Autodesk Inventor part; units mm, degrees
sketch "Skizze1" plane through (0, 0, 0) normal (0, 1, 0) x (-1, 0, 0)
  line L0 (34, -34) -> (-34, -34)
  line L1 (-34, -34) -> (-34, 34)
  line L2 (-34, 34) -> (34, 34)
  line L3 (34, 34) -> (34, -34)
  line L4 (0, -47.6) -> (0, 47.6)
  line L5 (47.6, 0) -> (-47.6, 0)
  point P0 (0, 0)
  dimension "d0" = 68
  dimension "d1" = 68
extrude "Extrusion1" add sketch "Skizze1" along normal blind 20
sketch "Skizze2" plane through (0, 20, 0) normal (0, 1, 0) x (1, 0, 0)
  line L0 (-30, 30) -> (30, 30)
  line L1 (30, 30) -> (30, -30)
  line L2 (30, -30) -> (-30, -30)
  line L3 (-30, -30) -> (-30, 30)
  line L4 (-47.6, 0) -> (47.6, 0)
  line L5 (0, 47.6) -> (0, -47.6)
  line L6 (-34, 34) -> (-34, -34)
  line L7 (34, -34) -> (34, 34)
  point P0 (0, 0)
  dimension "d4" = 60
  dimension "d5" = 60
  dimension "d6" = 4
  dimension "d7" = 4
extrude "Extrusion2" cut sketch "Skizze2" against normal blind 13
sketch "Skizze4" plane through (0, 0, 0) normal (0, -1, 0) x (1, 0, 0)
  line L0 (0, 12) -> (0, -12) construction
  line L1 (-2, 12) -> (-2, -12)
  line L2 (2, -12) -> (2, 12)
  arc A0 (2, 12) -> (-2, 12) centre (0, 12) ccw
  arc A1 (-2, -12) -> (2, -12) centre (0, -12) ccw
  line L3 (-47.6, 0) -> (47.6, 0)
  line L4 (12, 0) -> (-12, 0) construction
  line L5 (12, 2) -> (-12, 2)
  line L6 (-12, -2) -> (12, -2)
  arc A2 (12, -2) -> (12, 2) centre (12, 0) ccw
  arc A3 (-12, 2) -> (-12, -2) centre (-12, 0) ccw
  line L7 (0, -47.6) -> (0, 47.6)
  line L8 (-3.0851, 4.7663) -> (-2, 12)
  line L9 (3.0851, 4.7663) -> (2, 12)
  line L10 (-3.0851, -4.7663) -> (-2, -12)
  line L11 (3.0851, -4.7663) -> (2, -12)
  line L12 (-4.7663, 3.0851) -> (-12, 2)
  line L13 (-4.7663, -3.0851) -> (-12, -2)
  line L14 (4.7663, 3.0851) -> (12, 2)
  line L15 (4.7663, -3.0851) -> (12, -2)
  arc A4 (-4.7663, 3.0851) -> (-3.0851, 4.7663) centre (-5.0629, 5.0629) ccw
  arc A5 (3.0851, 4.7663) -> (4.7663, 3.0851) centre (5.0629, 5.0629) ccw
  arc A6 (4.7663, -3.0851) -> (3.0851, -4.7663) centre (5.0629, -5.0629) ccw
  arc A7 (-3.0851, -4.7663) -> (-4.7663, -3.0851) centre (-5.0629, -5.0629) ccw
  point P0 (0, 0)
  point P1 (0, 0)
  point P2 (0, 0)
  point P3 (-3.5, 2)
  point P4 (3.5, 2)
  point P5 (-3.5, -2)
  point P6 (3.5, -2)
  point P7 (-2, 3.5)
  point P8 (-2, -3.5)
  point P9 (2, 3.5)
  point P10 (2, -3.5)
  dimension "d30" = 4
  dimension "d31" = 24
  dimension "d32" = 2
  dimension "d33" = 4
  dimension "d34" = 24
  dimension "d35" = 2
  dimension "d36" = 2
extrude "Extrusion4" cut sketch "Skizze4" against normal blind 3
properties part number "Base"
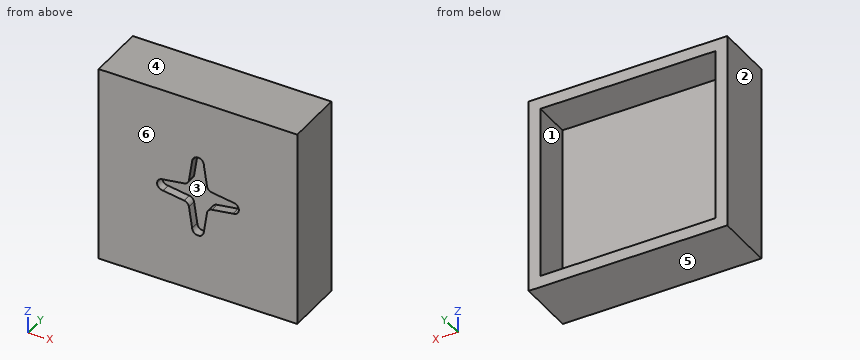
The listing builds one solid part. Answer for the finished solid, in the listing's coordinates (mm). Face numbers are marked on the shaded views. A direction names the side the tool comes from. Give positions to 0.01 mm unless a question says otherwise; leave off trailing zeros. Order: outer loops, then holes, each group sorted by start corner. A loop starts at its lowest first (then second) coordinate and runs counter-clockwise, first axis right, second up. Notation, with made-up numbers: (-39.75, 47) - (-0.75, 47) arc R21 ccw to (-0.75, 70) - close; hole circle Ø4 at (65, 61.25). An arc over 180 degrees is marked (long way). Answer in a Markdown table with one row per item. Add a question column.
Q1. The part is cut by section A-A (y = 12). Determine the outline of the cut face in (x, z), then the cut area to 3 significant figures.
Q2. The part is cut by section C-C (z = 1). Determine the outline of the cut face in (x, y), then the cut area to 3 significant figures.
Q3. Which of the six approach directions +Z, -Z, +X, -X, +Y, -Y give full straight-line access (tool end or side, diameter ignored) to the marked faces 1 and 2?
Q4. Given P1, Ø2, axis at x = -17.5, z = 6, coming from the -Y side; P2, Ø5, axis at x = 2.5, z = -15, coming from the +Y side, each flat-ended and moving along its own axis, determine where each tip first touches the part or whether it passes through.
Q5. For a pull along Z with two mould halves and no side action, classify the marked faces 3, 4, 5 and 6 as released by +Z, released by -Z, zero draft, split by the parting line, or undercut.
Q6. The part is cut by section D-D (x = -17). Determine the outline of the cut face in (y, z), then the cut area to 3 significant figures.
Q7. Find the intervals of material crossed by line 1 along Z through (x, y) = (16, 12.25); line 2 along Y through (x, z) = (-27.5, -20), in increasing order. Write a range as [from, to].
Q8. The part is cut by section B-B (x = 0). Determine the outline of the cut face in (y, z).
Determined:
| question | item | result |
|---|---|---|
| 1 | outline | (-34, -34) - (34, -34) - (34, 34) - (-34, 34) - close; hole (-30, -30) - (30, -30) - (30, 30) - (-30, 30) - close |
| 1 | area | 1,020 mm² |
| 2 | outline | (-34, 0) - (-13.73, 0) - (-13.73, 3) - (13.73, 3) - (13.73, 0) - (34, 0) - (34, 20) - (30, 20) - (30, 7) - (-30, 7) - (-30, 20) - (-34, 20) - close |
| 2 | area | 498 mm² |
| 3 | face 1 | +Y |
| 3 | face 2 | +Z, -Z, -X, +Y, -Y |
| 4 | P1 | stops at y = 0 |
| 4 | P2 | stops at y = 7 |
| 5 | face 3 | undercut |
| 5 | face 4 | released by +Z |
| 5 | face 5 | released by -Z |
| 5 | face 6 | zero draft |
| 6 | outline | (0, -34) - (20, -34) - (20, -30) - (7, -30) - (7, 30) - (20, 30) - (20, 34) - (0, 34) - close |
| 6 | area | 580 mm² |
| 7 | line 1 | z = [-34, -30], [30, 34] |
| 7 | line 2 | y = [0, 7] |
| 8 | outline | (0, -34) - (20, -34) - (20, -30) - (7, -30) - (7, 30) - (20, 30) - (20, 34) - (0, 34) - (0, 14) - (3, 14) - (3, -14) - (0, -14) - close |
